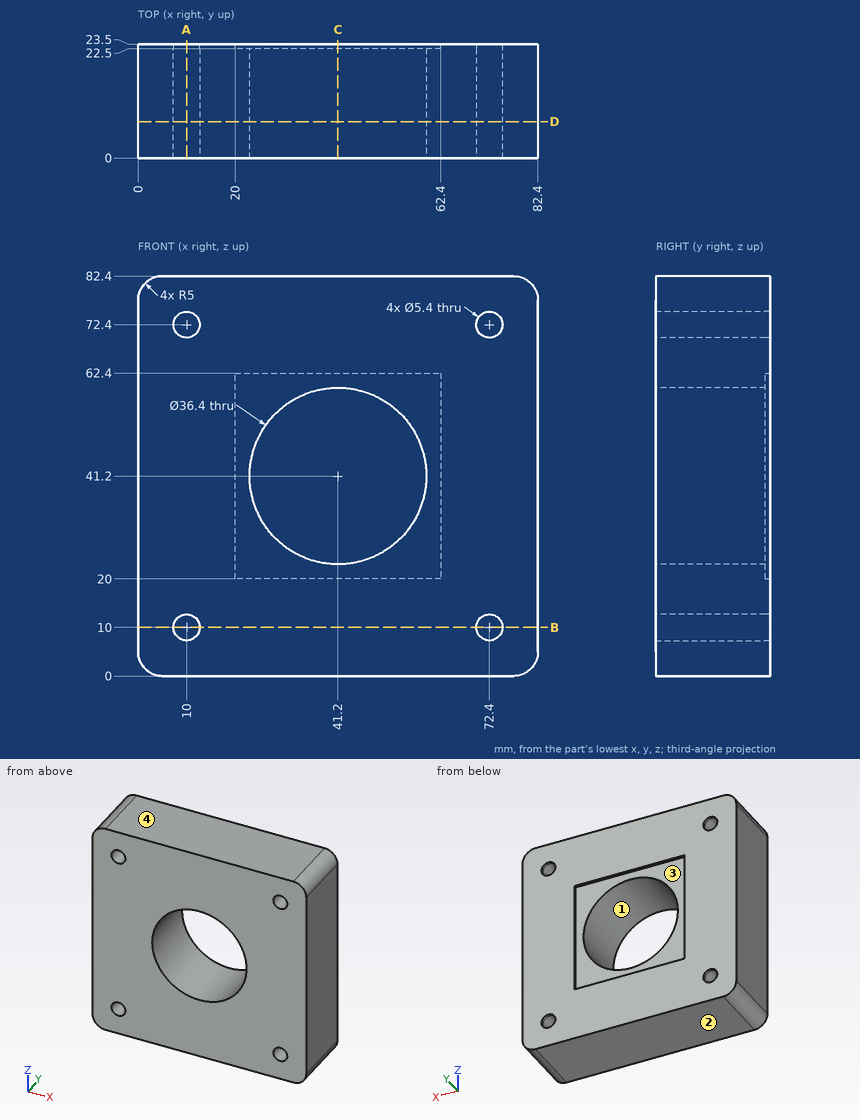
Part print with two shaded views. Sizes in mm from the minimum x, y, z corner. Round coordinates to 2 decimals unless told otherwise and drop trailing zeros. Order: outer loops, then holes, each group sorted by start corner. A loop starts at its lowest first (then second) coordinate and runs counter-clockwise, first axis right, second up. Notation, with made-up numbers: M 38,17.25 L 89,17.25 A8 cw 89,27.25 Z; hole C 18.25,47 d8. An arc over 180 degrees is marked long. Put each result on its own line as item: value. Start each with the question number.
1. Two-plate mould, pull along Z, no slides. Class the marked faces 1, 2, 3 and 4: +Z half, -Z half, draft (parallel to the pull), parting line (faces both ways), or undercut.
2. Slice it at B-B on z = 10. List the corners of the cut face in (x, y).
3. Slice it at D-D on y = 7.5. List the corners of the cut face in (x, z), then the cut area to 3 significant figures.
4. Slice it at A-A on x = 10. List the corners of the cut face in (y, z), then the cut area to 3 significant figures.
5. Slice it at C-C on x = 41.2. List the corners of the cut face in (y, z), then the cut area to 4 significant figures.
6. Drop a flat-ended pin along its axis: pin 1 (3 mm diameter, centred on x = 10, z = 72.4, fed in from -Y). Give the stop position or say it passes through.
7. Drill centre lines: probe 1 along Z at (x, y) = (72.4, 8.75); probe 2 along X at (y, z) = (7, 9). Where is each one in solid material? Low to high. Write a range as [from, to].
Findings:
1. face 1: undercut
1. face 2: -Z half
1. face 3: undercut
1. face 4: +Z half
2. outline: M 0,0 L 7.3,0 L 7.3,23.5 L 0,23.5 Z; M 12.7,0 L 69.7,0 L 69.7,23.5 L 12.7,23.5 Z; M 75.1,0 L 82.4,0 L 82.4,23.5 L 75.1,23.5 Z
3. outline: M 0,5 A5 ccw 5,0 L 77.4,0 A5 ccw 82.4,5 L 82.4,77.4 A5 ccw 77.4,82.4 L 5,82.4 A5 ccw 0,77.4 Z; hole C 10,10 d5.4; hole C 10,72.4 d5.4; hole C 41.2,41.2 d36.4; hole C 72.4,10 d5.4; hole C 72.4,72.4 d5.4
3. area: 5,640 mm2
4. outline: M 0,0 L 23.5,0 L 23.5,7.3 L 0,7.3 Z; M 0,12.7 L 23.5,12.7 L 23.5,69.7 L 0,69.7 Z; M 0,75.1 L 23.5,75.1 L 23.5,82.4 L 0,82.4 Z
4. area: 1,680 mm2
5. outline: M 0,0 L 23.5,0 L 23.5,20 L 22.5,20 L 22.5,23 L 0,23 Z; M 0,59.4 L 22.5,59.4 L 22.5,62.4 L 23.5,62.4 L 23.5,82.4 L 0,82.4 Z
5. area: 1,075 mm2
6. pin 1: through
7. probe 1: [0, 7.3], [12.7, 69.7], [75.1, 82.4]
7. probe 2: [0, 7.49], [12.51, 69.89], [74.91, 82.4]
